from build123d import *

# Parameters (mm, degrees)
BOSS_EXTRUDE1_DEPTH = 20


# Read off the part's stored shape, not the designer's step: Boss-Extrude1
with BuildPart() as part:
    # Boss-Extrude1 outline → Boss-Extrude1 (new body)
    with BuildSketch(Plane.XY):
        with BuildLine():
            add(Edge.make_bspline(
                [(88.876710402, -2.002586822), (88.9493666131852, -1.9299306111192516), (88.4625699978628, 0.4568259281849222), (87.07101235202, 4.161910300422061), (84.73052634724378, 8.45500011557144), (81.46452093002502, 12.839206368183609), (77.24103186625386, 17.00911709970944), (71.93195290896183, 20.803795803023178), (65.32925222978359, 24.158999559971143), (57.19621791696868, 27.06225253428082), (47.335015505133114, 29.51378107366912), (35.65507966429881, 31.49568730649157), (22.23010133812801, 32.95110874977801), (7.334610783619065, 33.77448207700359), (-8.545603873112306, 33.81339982544799), (-24.73176378798255, 32.88191945449804), (-40.39833431767832, 30.78455479775411), (-54.643270604282016, 27.349550583302506), (-66.57507756172521, 22.469411328020367), (-75.406248837651, 16.14602654328372), (-80.53941016190787, 8.537104820951011), (-83.39672891288393, -13.84522539502793), (-61.221940715805076, -15.925333234293028), (-49.587864737730854, -13.445940213401869), (-35.47439605280903, -11.347992129221693), (-35.474395138973044, 2.574753359034609), (-37.57234303482898, 13.63666157313359), (-90.59320738468432, 42.62648764825083), (6.865999341566411, 15.353169169956265), (21.55164652021018, 15.353165638104155), (23.649596419713923, 18.023280969032704), (59.69615314335737, 30.61096775758453), (54.355929072849776, 3.719095036640508), (59.696158438048975, -5.054145848334971), (52.257981621563104, -14.0181057250969), (13.350588262830351, -27.17796082242287), (84.68079572840632, -13.636666154662072), (87.92309673716264, -13.636662647508883), (91.16538011136153, -12.110882655992413), (91.16538105607023, -9.440767269492538), (89.0674336356561, -3.528369172562094), (88.876710402, -2.002586822)],
                knots=[0, 0, 0, 0, 0, 0, 0, 0, 0, 0, 0, 0, 0, 0, 0, 0, 0, 0, 0, 0, 0, 0, 1, 1, 1, 1, 1, 1, 1, 1, 1, 1, 1, 1, 1, 1, 1, 1, 1, 1, 1, 1, 2.62177057508421, 2.62177057508421, 2.62177057508421, 2.62177057508421, 2.62177057508421, 2.62177057508421, 2.62177057508421, 2.62177057508421, 2.62177057508421, 2.62177057508421, 2.62177057508421, 2.62177057508421, 2.62177057508421, 2.62177057508421, 2.62177057508421, 2.62177057508421, 2.62177057508421, 2.62177057508421, 2.62177057508421, 2.62177057508421, 2.62177057508421, 2.62177057508421], degree=21))
        make_face()
    extrude(amount=BOSS_EXTRUDE1_DEPTH)

    # Sketch7 → Revolve4 (revolve)
    with BuildSketch(Plane(origin=(2.6990032539533013, -13.65, 1.73e-15), x_dir=(1, 0, 0), z_dir=(0, 1, 0))):
        with BuildLine():
            Line((67.48143473107149, -30.87020769655964), (67.48143473107149, 9.44190425666576))
            ThreePointArc((67.48143473107149, 9.44190425666576), (47.32537875445879, -10.714151719946939), (67.48143473107149, -30.87020769655964))
        make_face()
    revolve4 = revolve(axis=Axis((70.1804379850248, -13.65, 30.87020769655964), (0, 0, -1)))

    # Mirror1: Revolve4 across plane
    add(revolve4.mirror(Plane(origin=(0, 0, 0), x_dir=(0, 0, 1), z_dir=(1, 0, 0))))


solid = part.part
The listing builds one solid part. Answer for the finished solid, in the listing's coordinates (mm). Coordinates: 2 decimals unless noted, no trailing zeros. Write each loop counter-clockwise with the first axis right and the second up, starting at its lowest first coordinate (ties: lowest second). Pieces come first, ordered by that corner, then holes. Notation, with made-up numbers: M -4.5,38 L 18.5,38 A11 cw 18.5,47 Z; hole C -3,49.25 d11. An arc over 180 degrees is marked long. Use one line per item in the form item = value.
Item 1: Given P1, Ø3, axis at x = -46, y = 25, coming from the +Z side; P2, Ø3, axis at x = 56, z = 0, coming from the -Y side; P3, Ø10, axis at x = -59, z = 1, coming from the -Y side, each flat-ended and moving along its own axis, determine where each tip first touches the part or whether it passes through.
Model answer:
P1 = 20
P2 = -25.54
P3 = -31.26
Item 2: Find the intervals of material crossed by probe 1 along X at (y, z) = (-14.5, 11); probe 2 along Z at (x, y) = (-8, 25); probe 3 along X at (y, z) = (-19, 19), in increasing order.
Model answer:
probe_1 = -90.32 to -50.04, 50.04 to 90.32
probe_2 = 0 to 20
probe_3 = -87.76 to -52.6, 52.6 to 87.76
Item 3: Find section A-A, the plane y = -25. Give the vertices of the cut face in (x, z).
Model answer:
outline = C -70.18,10.71 d33.31; C 70.18,10.71 d33.31
Item 4: Find section B-B, the plane z = 28.5. Give the vertices of the cut face in (x, y), plus the area to 3 significant figures.
Model answer:
outline = C -70.18,-13.65 d18.97; C 70.18,-13.65 d18.97
area = 565 mm2
